Can you work these out from the model? Positions are in its coordinate system, mm. Coordinates: 2 decimals unless noted, no trailing zeros. Order: outer loops, then holes, each group sorted by start corner. A loop starts at its lowest first (then second) coordinate and runs counter-clockwise, first axis right, second up. Notation, with made-up numbers: (84, 19.25) - (111, 19.25) arc R25 ccw to (111, 36.25) - close; hole circle Ø3 at (-17.75, 7.5). An arc over 180 degrees is marked (long way). Return JSON: item names as keys, results as strings. Group by question number.
1) If I drill on line 1 along X through (y, z) = (-34, -2); line 2 along X through (y, z) = (-33, -18.5); line 3 along Y through (x, z) = (-24, 1), over which ranges is the centre line in solid material (lowest first)?
2) Imagine slicing it at B-B (y = -35). Write out the boundary of the cut face in (x, z).
3) Imagine slicing it at C-C (y = -4). Write out the boundary of the cut face in (x, z), and give its area (3 significant figures).
4) Imagine slicing it at A-A (z = -19). Write out the boundary of the cut face in (x, y).
5) For pin 1 Ø1 at (y, z) = (-6.5, 28) entering from +X, with a flat end and sliding along its axis, tell me the tip position at first contact or that it passes through.
```python
from build123d import *

# Parameters (mm, degrees)
F0_W     = 58.5621017963
F0_H     = 77.0259462297
F1_DEPTH = 39.878
F2_R     = 7.971733183
F3_R     = 6.2062238441
F6_DEPTH = 0.762


# Not quite as in the source:
# - the program builds the solid bodies; features that only make, move or delete a surface that nothing else refers to are left out


with BuildPart() as f1:
    # F0 (on Front) → F1 (new body)
    with BuildSketch(Plane.XZ):
        with Locations((0.5595115945, 2.331295982)):
            Rectangle(F0_W, F0_H)
    extrude(amount=F1_DEPTH)

    # F2
    f2_edges = [f1.edges().sort_by_distance(p)[0] for p in [
        (29.840562, -39.878, 2.331296),
        (-28.721539, -39.878, 2.331296),
        (29.840562, 0, 2.331296),
        (-28.721539, 0, 2.331296),
    ]]
    fillet(f2_edges, radius=F2_R)

    # F3 (on face) → F6 (join)
    with BuildSketch(Plane.XY.offset(40.8442690969)):
        with BuildLine():
            Line((15.5188293097, -6.3193492971), (-17.34697557, -6.3193492971))
            ThreePointArc((-17.34697557, -6.3193492971), (-21.8371036305, -8.1792212365), (-23.69697557, -12.6693492971))
            Line((-23.69697557, -12.6693492971), (-23.69697557, -25.556266817))
            ThreePointArc((-23.69697557, -25.556266817), (-21.8371036305, -30.0463948776), (-17.34697557, -31.906266817))
            Line((-17.34697557, -31.906266817), (15.5188293097, -31.906266817))
            ThreePointArc((15.5188293097, -31.906266817), (20.0089573702, -30.0463948776), (21.8688293097, -25.556266817))
            Line((21.8688293097, -25.556266817), (21.8688293097, -12.6693492971))
            ThreePointArc((21.8688293097, -12.6693492971), (20.0089573702, -8.1792212365), (15.5188293097, -6.3193492971))
        make_face()
        Polygon((-8.0732123646, -19.3963646889), (-10.657480345, -23.8724481314), (-15.826016306, -23.8724481314), (-18.4102842865, -19.3963646889), (-15.826016306, -14.9202812463), (-10.657480345, -14.9202812463), align=None, mode=Mode.SUBTRACT)
        with Locations((8.9521687478, -19.2098617554)):
            Circle(F3_R, mode=Mode.SUBTRACT)
    extrude(amount=-F6_DEPTH)


solid = f1.part
```
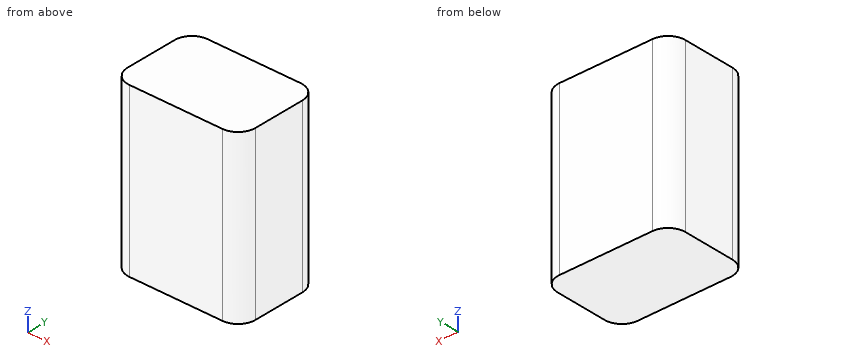
Calculated:
{
 "1": {"line 1": "-28.44 to 29.56", "line 2": "-28.65 to 29.77", "line 3": "-39.19 to -0.69"},
 "2": {"outline": "(-28.1, -36.18) - (29.22, -36.18) - (29.22, 40.84) - (-28.1, 40.84) - close"},
 "3": {"outline": "(-27.66, -36.18) - (28.78, -36.18) - (28.78, 40.84) - (-27.66, 40.84) - close", "area": "4,350 mm2"},
 "4": {"outline": "(-28.72, -31.91) arc R7.97 ccw to (-20.75, -39.88) - (21.87, -39.88) arc R7.97 ccw to (29.84, -31.91) - (29.84, -7.97) arc R7.97 ccw to (21.87, 0) - (-20.75, 0) arc R7.97 ccw to (-28.72, -7.97) - close"},
 "5": {"pin 1": "x = 29.78"}
}
